```python
from build123d import *

# Parameters (mm, degrees)
F0_R     = 2.5
F1_DEPTH = 7.5
F2_R     = 2.5
F4_DEPTH = 1
F6_W     = 0.5
F6_H     = 0.5
F7_DEPTH = 5.5


with BuildPart() as f1:
    # F0 (on Top) → F1 (new body)
    with BuildSketch(Plane.XY):
        Circle(F0_R)
    extrude(amount=F1_DEPTH)

    # F2
    f2_edges = [f1.edges().sort_by_distance(p)[0] for p in [
        (-2.5, 0, 7.5),
    ]]
    fillet(f2_edges, radius=F2_R)

    # F3 (on face) → F4 (join)
    with BuildSketch(Plane(origin=(0, 0, 0), x_dir=(1, 0, 0), z_dir=(0, 0, -1))):
        with BuildLine():
            Line((-1.2609520213, -2.5), (1.2609520213, -2.5))
            ThreePointArc((1.2609520213, -2.5), (0, 2.8), (-1.2609520213, -2.5))
        make_face()
    extrude(amount=F4_DEPTH)

    # F6 (on offset) → F7 (join)
    with BuildSketch(Plane(origin=(0, 0, -1), x_dir=(1, 0, 0), z_dir=(0, 0, -1))):
        with Locations((0.1509, 1.25)):
            Rectangle(F6_W, F6_H)
        with Locations((0.1509, -1.25)):
            Rectangle(F6_W, F6_H)
    extrude(amount=F7_DEPTH)


solid = f1.part
```
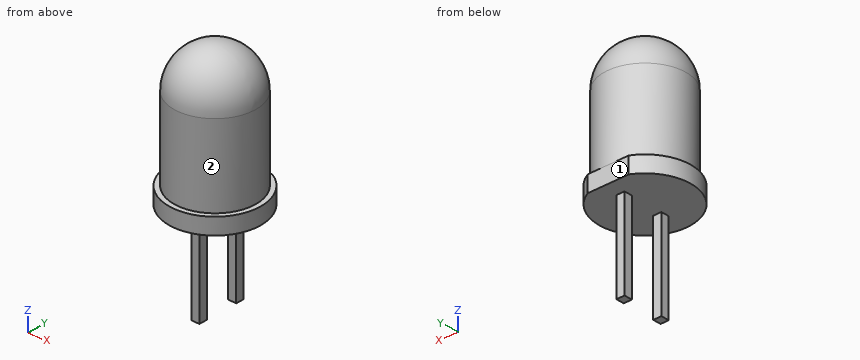
Geometry check sheet. Reference: the model listing, model coordinates, mm. Face numbers are marked on the shaded views. A direction names the side the tool comes from. Coordinates: 2 decimals unless noted, no trailing zeros. Order: outer loops, then holes, each group sorted by start corner. A loop starts at its lowest first (then second) coordinate and runs counter-clockwise, first axis right, second up.
Q1. Sectioned sample at A-A on z = -5.5. Record the cut outline in (x, y), and give its area (3 significant figures).
Reply:
outline: (-0.1, -1.5) - (0.4, -1.5) - (0.4, -1) - (-0.1, -1) - close; (-0.1, 1) - (0.4, 1) - (0.4, 1.5) - (-0.1, 1.5) - close
area: 0.500 mm2
Q2. Depth check by flat-ended pin: pin 1 Ø2 at (x, z) = (-1.5, 4.5) entering from +Y; pin 2 Ø2 at (x, y) = (2, -1.5) entering from +Z; pin 3 Ø1 at (y, z) = (1.5, 3.5) entering from -X. Enter the tip coordinate at first touch or a pass-through.
Reply:
pin 1: stops at y = 2.45
pin 2: stops at z = 7
pin 3: stops at x = -2.29
Q3. Sectioned sample at B-B on y = 0. Record the cut outline in (x, z), and give its area (3 significant figures).
Reply:
outline: (-2.8, -1) - (2.8, -1) - (2.8, 0) - (2.5, 0) - (2.5, 5) arc R2.5 ccw to (-2.5, 5) - (-2.5, 0) - (-2.8, 0) - close
area: 40.4 mm2
Q4. Sectioned sample at C-C on x = 0.85. Record the cut outline in (y, z), and give its area (3 significant figures).
Reply:
outline: (-2.67, -1) - (2.5, -1) - (2.5, 0) - (2.35, 0) - (2.35, 5) arc R2.35 ccw to (-2.35, 5) - (-2.35, 0) - (-2.67, 0) - close
area: 37.4 mm2
Q5. Tool access check on the marked faces 1 and 2. Record the directions out of +Z, -Z, +X, -X, +Y, -Y that give a thin tool (end or side, any length) a straight path to the whole face; none if there is none.
Reply:
face 1: +Z, -Z, +X, -X, +Y
face 2: +Z
Q6. Thickness scan on probe 1 along Z at (x, y) = (-0.05, -0.1); probe 2 along Z at (x, y) = (2, -1.85); probe 3 along X at (y, z) = (1.4, -5). Record the ranges inside material, lowest first.
Reply:
probe 1: z = -1 to 7.5
probe 2: z = -1 to 0
probe 3: x = -0.1 to 0.4
Q7. Sectioned sample at D-D on z = -0.5. Record the cut outline in (x, y).
Reply:
outline: (-1.26, 2.5) arc R2.8 ccw (long way) to (1.26, 2.5) - close
